CAD build for the part. Positions are in the model's coordinates, mm. Round coordinates to 2 decimals unless told otherwise and drop trailing zeros. Loops run counter-clockwise (first coordinate to the right, second up) from the corner with the lowest first, then second, coordinate; pieces in that order, holes last. Notation, with made-up numbers: M -16.75,31.25 L 27.25,31.25 A23 ccw 27.25,67.25 Z; hole C -34.75,68.5 d5. An arc over 180 degrees is marked long. Use one line per item in the form item = value.
Autodesk Fusion 360 part; units mm, degrees
sketch "Sketch1" plane through (0, 0, 0) normal (1, 0, 0) x (0, 1, 0)
  circle A0 centre (0, 0) radius 2.6
  circle A1 centre (122, 0) radius 2.6
  line L0 (-9, 7) -> (131, 7)
  line L1 (131, 7) -> (131, -7)
  line L2 (131, -7) -> (-9, -7)
  line L3 (-9, -7) -> (-9, 7)
  dimension "d1" = 5.2
  dimension "d3" = 5.2
extrude "Extrude1" add sketch "Sketch1" along normal mid plane 16
1. Cut at A-A on y = 122. Write the cut outline in (x, z).
Completed:
outline = M -8,-7 L 8,-7 L 8,-2.6 L -8,-2.6 Z; M -8,2.6 L 8,2.6 L 8,7 L -8,7 Z
2. Cut at C-C on x = 6.75. Write the cut outline in (y, z), and give its area (3 significant figures).
Completed:
outline = M -9,-7 L 131,-7 L 131,7 L -9,7 Z; hole C 0,0 d5.2; hole C 122,0 d5.2
area = 1,920 mm2
3. Cut at B-B on z = 0. Write the cut outline in (x, y), and give its area (3 significant figures).
Completed:
outline = M -8,-9 L 8,-9 L 8,-2.6 L -8,-2.6 Z; M -8,2.6 L 8,2.6 L 8,119.4 L -8,119.4 Z; M -8,124.6 L 8,124.6 L 8,131 L -8,131 Z
area = 2,070 mm2
4. Pull direction Y, two halves, no side cores. Call faces 1 (the face through (0, 60, 7)), 2 (the face through (0, 131, 0)), 3 (the face through (-0.11, 124.48, -0.78)): +Y half, -Y half, draft (parallel to the pull), parting line (faces both ways), or undercut.
Completed:
face_1 = draft
face_2 = +Y half
face_3 = undercut
5. Cut at D-D on y = 1. Write the cut outline in (x, z), and give its area (3 significant figures).
Completed:
outline = M -8,-7 L 8,-7 L 8,-2.4 L -8,-2.4 Z; M -8,2.4 L 8,2.4 L 8,7 L -8,7 Z
area = 147 mm2
6. Probe line 1 along Y through (x, z) = (5, -0.25); line 2 along Z through (x, y) = (3.5, 0); line 3 along Y through (x, z) = (1.25, -1.25). List the from-to ranges inside material, lowest first. Write a range as from..to.
Completed:
line_1 = -9..-2.59, 2.59..119.41, 124.59..131
line_2 = -7..-2.6, 2.6..7
line_3 = -9..-2.28, 2.28..119.72, 124.28..131
